Check sheet for the drawn part. Datum: minimum x, y, z corner. Units: mm. A direction names the side the tool comes from. Coordinates: 2 decimals unless noted, no trailing zeros. Order: outer loops, then holes, each group sorted by start corner. A loop starts at its lowest first (then second) coordinate and runs counter-clockwise, first axis right, second up. Notation, with made-up numbers: M 35,-8.75 L 42,-8.75 A14 ccw 42,-0.75 Z; hole C -1,2.5 d3. An arc over 180 degrees is marked long. Answer in a Markdown table with one row per item. Add a question column.
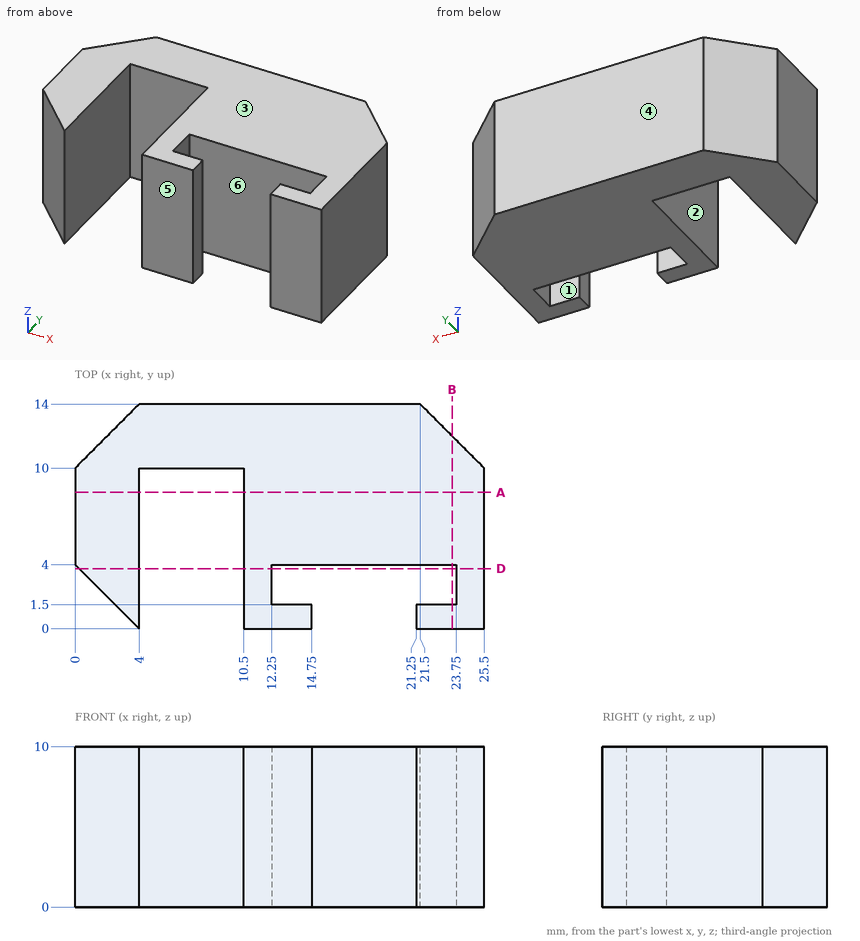
1. Go/stop test with flat-tipped pins: pin 1 Ø2 at (x, y) = (6.5, 1.5) entering from +Z; pin 2 Ø1.7 at (y, z) = (1, 3.5) entering from -X; pin 3 Ø1.2 at (y, z) = (2.5, 7) entering from -X; pin 4 Ø2 at (x, z) = (5.5, 3) entering from -Y. Record where each tip stops, or that it passes through.
2. Release check for a two-part mould opening along Y. For the marked faces 4, 5 and 6 record: released by +Y, released by -Y, zero draft, split by the parting line, or undercut.
3. Section check A-A on y = 8.5. Enter the section's corners in (x, z), then the cut area to 3 significant figures.
4. Section check D-D on y = 3.75. Enter the section's corners in (x, z).
5. Section check B-B on x = 23.5. Enter the section's corners in (y, z).
6. Scan lines: line 1 (X direction, y = 9, z = 9.25); line 2 (Y direction, x = 14, z = 7); line 3 (X direction, y = 1, z = 5). Record each from-to range of solid material in increasing order.
7. Set-up check for the marked faces 1, 2 and 3: record each of +Z, -Z, +X, -X, +Y, -Y from which the full face is reachable in a straight line by a thin tool's end or side.
Result sheet:
| question | item | result |
|---|---|---|
| 1 | pin 1 | through |
| 1 | pin 2 | x = 2.15 |
| 1 | pin 3 | x = 0.9 |
| 1 | pin 4 | y = 10 |
| 2 | face 4 | released by +Y |
| 2 | face 5 | released by -Y |
| 2 | face 6 | undercut |
| 3 | outline | M 0,0 L 4,0 L 4,10 L 0,10 Z; M 10.5,0 L 25.5,0 L 25.5,10 L 10.5,10 Z |
| 3 | area | 190 mm^2 |
| 4 | outline | M 0.25,0 L 4,0 L 4,10 L 0.25,10 Z; M 10.5,0 L 12.25,0 L 12.25,10 L 10.5,10 Z; M 23.75,0 L 25.5,0 L 25.5,10 L 23.75,10 Z |
| 5 | outline | M 0,0 L 1.5,0 L 1.5,10 L 0,10 Z; M 4,0 L 12,0 L 12,10 L 4,10 Z |
| 6 | line 1 | 0 to 4, 10.5 to 25.5 |
| 6 | line 2 | 0 to 1.5, 4 to 14 |
| 6 | line 3 | 3 to 4, 10.5 to 14.75, 21.25 to 25.5 |
| 7 | face 1 | +Z, -Z |
| 7 | face 2 | +Z, -Z, -Y |
| 7 | face 3 | +Z, +X, -X, +Y, -Y |
